```python
from build123d import *

# Parameters (mm, degrees)
SKETCH008_W     = 18
SKETCH008_H     = 5
PAD008_DEPTH    = 4
SKETCH010_W     = 9.9
SKETCH010_H     = 1.99
PAD009_DEPTH    = 4
POCKET006_DEPTH = 5
SKETCH014_W     = 12
SKETCH014_H     = 1.8
PAD011_DEPTH    = 5


with BuildPart() as part:
    # Sketch008 → Pad008 (new body)
    with BuildSketch(Plane(origin=(0, -10.4875, 0), x_dir=(-1, 0, 0), z_dir=(0, 1, 0))):
        with Locations((0, -1.5)):
            Rectangle(SKETCH008_W, SKETCH008_H)
    extrude(amount=-PAD008_DEPTH)

    # Sketch010 → Pad009 (new body)
    with BuildSketch(Plane(origin=(0, -10.4875, 1), x_dir=(1, 0, 0), z_dir=(0, 0, 1))):
        with Locations((0, -2.995)):
            Rectangle(SKETCH010_W, SKETCH010_H)
    extrude(amount=PAD009_DEPTH)

    # Sketch013 → Pocket006 (cut)
    with BuildSketch(Plane(origin=(0, -12.4875, 0), x_dir=(-1, 0, 0), z_dir=(0, 1, 0))):
        with BuildLine():
            ThreePointArc((2, 3), (1.5, 2.5), (2, 2))
            Line((2, 2), (4, 2))
            ThreePointArc((4, 2), (4.5, 2.5), (4, 3))
            Line((2, 3), (4, 3))
        make_face()
        with BuildLine():
            ThreePointArc((-4, 3), (-4.5, 2.5), (-4, 2))
            Line((-4, 2), (-2, 2))
            ThreePointArc((-2, 2), (-1.5, 2.5), (-2, 3))
            Line((-4, 3), (-2, 3))
        make_face()
    extrude(amount=-POCKET006_DEPTH, mode=Mode.SUBTRACT)

    # Sketch014 → Pad011 (new body)
    with BuildSketch(Plane(origin=(0, -14.4875, 0), x_dir=(-1, 0, 0), z_dir=(0, -1, 0))):
        with Locations((0, 3.1)):
            Rectangle(SKETCH014_W, SKETCH014_H)
    extrude(amount=PAD011_DEPTH)


solid = part.part
```
Input: part model. Units: mm. Frame: model coordinates. A direction names the side the tool comes from. Coordinates: 2 decimals unless noted, no trailing zeros. Loops run counter-clockwise (first coordinate to the right, second up) from the corner with the lowest first, then second, coordinate; pieces in that order, holes last. Notation, with made-up numbers: (14, 79.5) - (46, 79.5) arc R31 cw to (46, 103.5) - close; hole circle Ø3 at (-37.75, 11). An arc over 180 degrees is marked (long way). Answer in a Markdown table with one row per item.
(1) Pin query (flat end, axial travel): P1, Ø0.9, axis at y = -18, z = -3, coming from the +X side; P2, Ø4, axis at x = -1.5, y = -18, coming from the +Z side; P3, Ø1, axis at y = -13.5, z = 3, coming from the -X side. Return the tip coordinate at first contact, or that it passes through.
Model answer:
| item | result |
|---|---|
| P1 | stops at x = 6 |
| P2 | stops at z = -2.2 |
| P3 | stops at x = -4.95 |
(2) Cut plane A-A on z = 2.5. Output: boundary loops of the cut face in (x, y).
Model answer:
| item | result |
|---|---|
| outline | (-4.95, -14.48) - (-4.5, -14.48) - (-4.5, -12.49) - (-4.95, -12.49) - close; (-1.5, -14.48) - (1.5, -14.48) - (1.5, -12.49) - (-1.5, -12.49) - close; (4.5, -14.48) - (4.95, -14.48) - (4.95, -12.49) - (4.5, -12.49) - close |
(3) Mould query, pull axis Z, two halves, no side actions, for faces 5 (the face through (-1.5, -13.5, 2.5)), 6 (the face through (0, -15, -4)), 7 (the face through (3, -13, 3)), 8 (the face through (-9, -12, -2)). Classes: pulls with the +Z half, pulls with the -Z half, needs draft (parallel to the pull), parting line crosses it, or undercut.
Model answer:
| item | result |
|---|---|
| face 5 | undercut |
| face 6 | pulls with the -Z half |
| face 7 | undercut |
| face 8 | needs draft |
(4) Cut plane C-C on y = -14.25. Output: boundary loops of the cut face in (x, z), plus the area to 3 significant figures.
Model answer:
| item | result |
|---|---|
| outline | (-9, -4) - (9, -4) - (9, 1) - (4.95, 1) - (4.95, 5) - (-4.95, 5) - (-4.95, 1) - (-9, 1) - close; hole (-4, 2) - (-2, 2) arc R0.5 ccw to (-2, 3) - (-4, 3) arc R0.5 ccw to start; hole (2, 2) - (4, 2) arc R0.5 ccw to (4, 3) - (2, 3) arc R0.5 ccw to start |
| area | 124 mm² |
(5) Set-up query: faces 1 (the face through (4.5, -13.5, 2.5)), 2 (the face through (-4.95, -13, 3)), 3 (the face through (0, -12.488, 3)), 4 (the face through (-6, -17, -3)). Return all of +Z, -Z, +X, -X, +Y, -Y with unobstructed straight access to the full face (end or side cutting, diameter ignored); none if empty.
Model answer:
| item | result |
|---|---|
| face 1 | +Y, -Y |
| face 2 | +Z, -X, +Y, -Y |
| face 3 | +Z, +X, -X, +Y |
| face 4 | +Z, -Z, -X, -Y |
(6) Material intervals for L1, parallel to X at y = -13.75, z = 2.25; L2, parallel to Y at x = 4.25, z = 0.75; L3, parallel to Z at x = 4.5, y = -17.5, sorted ascending. Write a range as from..to.
Model answer:
| item | result |
|---|---|
| L1 | x = -4.95..-4.43, -1.57..1.57, 4.43..4.95 |
| L2 | y = -14.49..-10.49 |
| L3 | z = -4..-2.2 |
